Build history of the part. All positions in model axes, mm. A direction names the side the tool comes from. Give positions to 0.01 mm unless a question says otherwise; leave off trailing zeros. Loops run counter-clockwise (first coordinate to the right, second up) from the corner with the lowest first, then second, coordinate; pieces in that order, holes last. Notation, with made-up numbers: (52.25, 74.5) -> (88.25, 74.5) arc R22 cw to (88.25, 91.5) -> close; hole circle Ø3 at (-7.5, -17). An arc over 180 degrees is marked (long way). One line per question, with ' | ' between items. Start each with the question number.
(1) Slice it at C-C, the plane y = 3.5. Write the cut outline in (x, z) (3 decimals), then the cut area to 3 significant figures.
(2) Flat gauge pins, fed straight in: pin 1 Ø6.5 at (y, z) = (-2.06, -8.5) entering from +X; pin 2 Ø0.8 at (x, z) = (51, -75.5) entering from +Y; pin 3 Ø10 at (y, z) = (-8, -21) entering from -X; pin 4 Ø3 at (y, z) = (5, -44.5) entering from +X. Where does each tip first touch, or does it go through?
(3) Slice it at B-B, the plane z = -44.5. Give the number of separate pieces and of enclosed holes in the cut face, then the cut area to 3 significant figures.
(4) Drill centre lines: L1, parallel to Y at x = 49.9, z = -98; L2, parallel to Z at x = 50, y = -2 (3 decimals); L3, parallel to X at y = 5, z = -10. Where is each one in solid material? Low to high. Write a range as from..to.
(5) 3-axis set-ups, long thin cutter, end or side, ignore diameter. For faces 4 (the face through (-10.04, 20.9, -20.33)), 5 (the face through (51, 7.656, -45)), 6 (the face through (51, -9.06, -95)): which of +Z, -Z, +X, -X, +Y, -Y reach the whole face in a straight line?
(6) Mould opens along Y. For faces 1 (the face through (-4, 20, -109)), 2 (the face through (51, -8.81, -80)), 3 (the face through (-51, -19.63, -101)) say: pulls with the +Y half, pulls with the -Y half, needs draft (parallel to the pull), parting line crosses it, or undercut.
Autodesk Inventor part; units mm, degrees
ref_plane "Work Plane1" through (-49.5, -19.63, -109) normal (0, 0, -1) x (0, 1, 0)
ref_plane "Work Plane2" through (-47.0185, 3.2145, -3.5) normal (1, 0, 0) x (0, 1, 0)
ref_plane "YZ Plane" through (0, 0, 0) normal (1, 0, 0) x (0, 1, 0)
sketch "Sketch1" plane through (0, 0, 0) normal (0, 0, 1) x (1, 0, 0)
  line L0 (47.5, 19.63) -> (-47.5, 19.63)
  arc A0 (-47.5, 19.63) -> (-49.5, 17.63) centre (-47.5, 17.63) ccw
  line L1 (-49.5, 17.63) -> (-49.5, -19.63)
  line L2 (49.5, -19.63) -> (49.5, 17.63)
  arc A1 (49.5, 17.63) -> (47.5, 19.63) centre (47.5, 17.63) ccw
  line L3 (-49.5, -19.63) -> (-52, -19.63)
  line L4 (-52, -19.63) -> (-52, 20.13)
  line L5 (-50, 22.13) -> (50, 22.13)
  line L6 (52, 20.13) -> (52, -19.63)
  line L7 (52, -19.63) -> (49.5, -19.63)
  arc A2 (-50, 22.13) -> (-52, 20.13) centre (-50, 20.13) ccw
  arc A3 (52, 20.13) -> (50, 22.13) centre (50, 20.13) ccw
  dimension "d0" = 2.5
  dimension "d1" = 2.5
  dimension "d2" = 2.5
  dimension "d3" = 2
ref_plane "Work Plane1" through (-49.5, -19.63, -109) normal (0, 0, -1) x (0, 1, 0)
extrude "Extrusion1" add sketch "Sketch1" against normal up to surface (109 mm away)
sketch "Sketch2" plane through (-50, 22.13, 0) normal (0, 1, 0) x (1, 0, 0)
  circle A0 centre (39.65, 50.5) radius 18.5 construction
  line L0 (58.85, 79.4) -> (20.45, 79.4) construction
  line L1 (20.45, 79.4) -> (20.45, 21.6) construction
  line L2 (58.85, 21.6) -> (58.85, 79.4) construction
  line L3 (20.45, 21.6) -> (58.85, 21.6) construction
  line L4 (20.15, 23.6) -> (20.15, 77.4) construction
  line L5 (59.15, 77.4) -> (59.15, 23.6) construction
  line L6 (20.15, 21.6) -> (59.15, 21.6) construction
  line L7 (59.15, 79.4) -> (20.15, 79.4) construction
  line L8 (20.15, 21.6) -> (59.15, 21.6)
  line L9 (59.15, 21.6) -> (59.15, 79.4)
  line L10 (59.15, 79.4) -> (20.15, 79.4)
  line L11 (20.15, 79.4) -> (20.15, 21.6)
  line L12 (59.65, 79.4) -> (19.65, 79.4)
  line L13 (19.65, 79.4) -> (19.65, 21.6)
  line L14 (19.65, 21.6) -> (59.65, 21.6)
  line L15 (59.65, 21.6) -> (59.65, 79.4)
  point P0 (50, 0)
  point P1 (59.65, 50.5)
  point P2 (59.15, 79.4)
  dimension "d43" = 40
  dimension "d44" = 39
  dimension "d45" = 0.5
extrude "Extrusion2" cut sketch "Sketch2" against normal up to surface (2.5 mm away)
chamfer "Chamfer1" distance 2.5 angle 45 4 edges at (-10.35, 22.13, -79.4) (-30.35, 22.13, -50.5) (9.65, 22.13, -50.5) (-10.35, 22.13, -21.6)
sketch "Sketch3" plane through (-52, -19.63, 0) normal (-1, 0, 0) x (0, 0, 1)
  line L0 (-94, 9.5) -> (-94, 37.26)
  arc A0 (-92, 39.26) -> (-94, 37.26) centre (-92, 37.26) ccw
  line L1 (-92, 39.26) -> (-17, 39.26)
  arc A1 (-15, 37.26) -> (-17, 39.26) centre (-17, 37.26) ccw
  line L2 (-15, 37.26) -> (-15, 9.5)
  line L3 (-94, 9.5) -> (-94, 0)
  line L4 (0, 0) -> (-109, 0) construction
  line L5 (-15, 9.5) -> (-15, 0)
  line L6 (-94, 0) -> (-15, 0)
  circle A2 centre (-98, 6.25) radius 1.5 construction
  circle A3 centre (-11, 6.25) radius 1.5 construction
  circle A4 centre (-98, 6.25) radius 1.75
  circle A5 centre (-11, 6.25) radius 1.75
  point P0 (0, 19.63)
  dimension "d13" = 3.5
  dimension "d14" = 3.5
ref_plane "Work Plane2" through (-47.0185, 3.2145, -3.5) normal (1, 0, 0) x (0, 1, 0)
extrude "Extrusion3" cut sketch "Sketch3" against normal up to surface (4.9815 mm away)
sketch "Sketch4" plane through (52, -19.63, 0) normal (1, 0, 0) x (0, 0, -1)
  circle A0 centre (98, 6.25) radius 1.5 construction
  circle A1 centre (11, 6.25) radius 1.5 construction
  arc A2 (72.9, 14.47) -> (72.9168, 14.38) centre (73.1508, 14.4702) ccw construction
  line L0 (72.9, 16.76) -> (72.9, 14.47) construction
  line L1 (72.9, 16.76) -> (72.9, 18.76) construction
  line L2 (72.9, 22.14) -> (72.9, 18.76) construction
  arc A3 (73.15, 22.39) -> (72.9, 22.14) centre (73.15, 22.14) ccw construction
  line L3 (73.15, 22.39) -> (85.55, 22.39) construction
  arc A4 (85.8, 22.14) -> (85.55, 22.39) centre (85.55, 22.14) ccw construction
  line L4 (85.8, 22.14) -> (85.8, 18.76) construction
  line L5 (85.8, 18.76) -> (85.8, 16.76) construction
  line L6 (85.8, 16.76) -> (85.8, 14.47) construction
  arc A5 (85.7832, 14.38) -> (85.8, 14.47) centre (85.5492, 14.4702) ccw construction
  line L7 (85.7832, 14.38) -> (86.5, 14.38) construction
  line L8 (86.5, 14.38) -> (86.5, 12.03) construction
  line L9 (81.88, 12.03) -> (86.5, 12.03) construction
  line L10 (81.88, 12.03) -> (81.88, 11.42) construction
  line L11 (81.88, 11.42) -> (86.45, 11.42) construction
  line L12 (87.2, 11.42) -> (86.45, 11.42) construction
  line L13 (87.2, 24.47) -> (87.2, 11.42) construction
  line L14 (87.2, 24.52) -> (87.2, 24.47) construction
  line L15 (87.2, 24.52) -> (71.7, 24.52) construction
  line L16 (71.7, 24.52) -> (71.7, 24.47) construction
  line L17 (71.7, 24.47) -> (71.7, 11.42) construction
  line L18 (71.7, 11.42) -> (72.45, 11.42) construction
  line L19 (72.45, 11.42) -> (76.82, 11.42) construction
  line L20 (76.82, 12.03) -> (76.82, 11.42) construction
  line L21 (72.3, 12.03) -> (76.82, 12.03) construction
  line L22 (72.3, 14.38) -> (72.3, 12.03) construction
  line L23 (72.3, 14.38) -> (72.9168, 14.38) construction
  line L24 (68.675, 20.9412) -> (68.975, 20.9412) construction
  line L25 (68.975, 20.9412) -> (68.975, 26.4362) construction
  arc A6 (68.975, 26.4362) -> (68.375, 27.0362) centre (68.375, 26.4362) ccw construction
  line L26 (68.375, 27.0362) -> (55.825, 27.0362) construction
  arc A7 (55.825, 27.0362) -> (55.225, 26.4362) centre (55.825, 26.4362) ccw construction
  line L27 (55.225, 26.4362) -> (55.225, 20.9412) construction
  line L28 (55.225, 20.9412) -> (55.525, 20.9412) construction
  line L29 (55.525, 26.4362) -> (55.525, 20.9412) construction
  arc A8 (55.825, 26.7362) -> (55.525, 26.4362) centre (55.825, 26.4362) ccw construction
  line L30 (68.375, 26.7362) -> (55.825, 26.7362) construction
  arc A9 (68.675, 26.4362) -> (68.375, 26.7362) centre (68.375, 26.4362) ccw construction
  line L31 (68.675, 26.4362) -> (68.675, 20.9412) construction
  line L32 (51.675, 20.9412) -> (51.975, 20.9412) construction
  line L33 (51.975, 20.9412) -> (51.975, 26.4362) construction
  arc A10 (51.975, 26.4362) -> (51.375, 27.0362) centre (51.375, 26.4362) ccw construction
  line L34 (51.375, 27.0362) -> (38.825, 27.0362) construction
  arc A11 (38.825, 27.0362) -> (38.225, 26.4362) centre (38.825, 26.4362) ccw construction
  line L35 (38.225, 26.4362) -> (38.225, 20.9412) construction
  line L36 (38.225, 20.9412) -> (38.525, 20.9412) construction
  line L37 (38.525, 26.4362) -> (38.525, 20.9412) construction
  arc A12 (38.825, 26.7362) -> (38.525, 26.4362) centre (38.825, 26.4362) ccw construction
  line L38 (51.375, 26.7362) -> (38.825, 26.7362) construction
  arc A13 (51.675, 26.4362) -> (51.375, 26.7362) centre (51.375, 26.4362) ccw construction
  line L39 (51.675, 26.4362) -> (51.675, 20.9412) construction
  line L40 (34.7, 28.373) -> (34.7, 24.4594) construction
  line L41 (30.79, 29.2462) -> (33.9, 29.2462) construction
  line L42 (18.6, 29.2462) -> (21.71, 29.2462) construction
  line L43 (17.8, 25.8062) -> (17.8, 28.4462) construction
  line L44 (17.8, 12.6412) -> (17.8, 25.8412) construction
  line L45 (34.7, 12.6412) -> (34.7, 24.4412) construction
  line L46 (3.1, 11.07) -> (101.9, 11.07) construction
  circle A14 centre (8.5, 17.57) radius 4
  circle A15 centre (11, 6.25) radius 1.75
  circle A16 centre (98, 6.25) radius 1.75
  line L47 (17.55, 29.4962) -> (34.95, 29.4962)
  line L48 (34.95, 29.4962) -> (34.95, 10.82)
  line L49 (34.95, 10.82) -> (17.55, 10.82)
  line L50 (17.55, 10.82) -> (17.55, 29.4962)
  line L51 (37.975, 27.2862) -> (52.225, 27.2862)
  line L52 (52.225, 27.2862) -> (52.225, 10.82)
  line L53 (52.225, 10.82) -> (37.975, 10.82)
  line L54 (37.975, 10.82) -> (37.975, 27.2862)
  line L55 (54.975, 27.2862) -> (69.225, 27.2862)
  line L56 (69.225, 27.2862) -> (69.225, 10.82)
  line L57 (69.225, 10.82) -> (54.975, 10.82)
  line L58 (54.975, 10.82) -> (54.975, 27.2862)
  line L59 (71.45, 24.72) -> (87.45, 24.72)
  line L60 (87.45, 24.72) -> (87.45, 10.82)
  line L61 (87.45, 10.82) -> (71.45, 10.82)
  line L62 (71.45, 10.82) -> (71.45, 24.72)
  line L63 (90.5, 13.2962) -> (90.5, 12.7462) construction
  line L64 (91.35, 13.7962) -> (91, 13.7962) construction
  line L65 (98, 13.7962) -> (97.6, 13.7962) construction
  line L66 (98.5, 13.2962) -> (98.5, 12.7462) construction
  line L67 (89.75, 14.2962) -> (99.25, 14.2962)
  line L68 (99.25, 14.2962) -> (99.25, 10.57)
  line L69 (99.25, 10.57) -> (89.75, 10.57)
  line L70 (89.75, 10.57) -> (89.75, 14.2962)
  line L71 (71.7, 24.47) -> (87.2, 24.47) construction
  line L72 (87.2, 24.47) -> (87.2, 11.07) construction
  line L73 (87.2, 11.07) -> (71.7, 11.07) construction
  line L74 (71.7, 11.07) -> (71.7, 24.47) construction
  circle A17 centre (8.5, 17.57) radius 3.2
  point P0 (0, 19.63)
  point P1 (17.8, 27.1262)
  point P2 (68.975, 23.6887)
  point P3 (91.175, 13.7962)
  point P4 (90.5, 13.0212)
  point P5 (98.5, 13.0212)
  dimension "d15" = 8
  dimension "d16" = 3.5
  dimension "d17" = 3.5
  dimension "d18" = 0.25
  dimension "d19" = 0.25
  dimension "d20" = 0.25
  dimension "d21" = 0.25
  dimension "d22" = 0.25
  dimension "d23" = 0.25
  dimension "d24" = 0.25
  dimension "d25" = 0.25
  dimension "d26" = 0.25
  dimension "d27" = 0.25
  dimension "d28" = 0.25
  dimension "d29" = 0.25
  dimension "d30" = 0.25
  dimension "d31" = 0.25
  dimension "d32" = 0.25
  dimension "d33" = 0.25
  dimension "d34" = 0.5
  dimension "d35" = 0.5
  dimension "d36" = 0.75
  dimension "d37" = 0.75
extrude "Extrusion4" cut sketch "Sketch4" against normal up to surface (2.5 mm away) contours A14 | A15 | A16 | L47 L48 L49 L50 | L51 L52 L53 L54 | L55 L56 L57 L58 | L59 L60 L61 L62 | L67 L68 L69 L70 | A17
chamfer "Chamfer2" distance 2 angle 45 4 edges at (52, -13.38, -9.25) (52, -13.38, -96.25) (-52, -13.38, -99.75) (-52, -13.38, -12.75)
equation "\"d1\" = d0"
equation "\"d2\" = d0"
equation "\"d45\" = -0.5 * d44 + 0.5 * d43"
equation "\"d14\" = d13"
equation "\"d17\" = d16"
equation "\"d20\" = d18"
equation "\"d21\" = d18"
equation "\"d22\" = d19"
equation "\"d23\" = d20"
equation "\"d24\" = d23"
equation "\"d25\" = d24"
equation "\"d26\" = d24"
equation "\"d28\" = d26"
equation "\"d29\" = d25"
equation "\"d30\" = d29"
equation "\"d31\" = d27"
equation "\"d32\" = d31"
equation "\"d33\" = d31"
equation "\"d34\" = d35"
properties part number "Shroud Top"
Final values:
1) outline: (-52, -109) -> (-49.5, -109) -> (-49.5, -94) -> (-52, -94) -> close; (-52, -15) -> (-49.5, -15) -> (-49.5, 0) -> (-52, 0) -> close; (49.5, -109) -> (52, -109) -> (52, -87.45) -> (49.5, -87.45) -> close; (49.5, -71.45) -> (52, -71.45) -> (52, -69.225) -> (49.5, -69.225) -> close; (49.5, -54.975) -> (52, -54.975) -> (52, -52.225) -> (49.5, -52.225) -> close; (49.5, -37.975) -> (52, -37.975) -> (52, -34.95) -> (49.5, -34.95) -> close; (49.5, -17.55) -> (52, -17.55) -> (52, 0) -> (49.5, 0) -> close | area: 193 mm2
2) pin 1: x = -49.5 | pin 2: y = 22.04 | pin 3: x = 49.5 | pin 4: through
3) separate pieces: 3 | enclosed holes: 0 | area: 210 mm2
4) L1: -19.63..-15.13, -11.63..-9.06, -5.33..22.13 | L2: -109..-87.45, -71.45..-69.225, -54.975..-52.225, -37.975..-34.95, -17.55..-12.5, -4.5..0 | L3: -52..-49.5, 49.5..52
5) face 4: +Y | face 5: +X, -X | face 6: +X
6) face 1: needs draft | face 2: undercut | face 3: pulls with the -Y half
